from build123d import *

# Parameters (mm, degrees)
CROQUIS1_R              = 1.75
SALIENTE_EXTRUIR1_DEPTH = 2
CROQUIS2_R              = 1.75
SALIENTE_EXTRUIR2_DEPTH = 64
CORTAR_EXTRUIR1_DEPTH   = 62
REDONDEO1_R             = 2
CORTAR_EXTRUIR2_REACH   = 56
CROQUIS5_W              = 10.1
CROQUIS5_H              = 56.5


with BuildPart() as part:
    # Croquis1 → Saliente-Extruir1 (new body)
    with BuildSketch(Plane(origin=(0, 89.4998128, 0), x_dir=(1, 0, 0), z_dir=(0, 1, 0))):
        with BuildLine():
            Line((-45.118250968, 6.084971867), (-5.118250968, 6.084971867))
            ThreePointArc((-5.118250968, 6.084971867), (-0.1685035, 8.135224399), (1.881749032, 13.084971867))
            Line((1.881749032, 13.084971867), (1.881749032, 43.084971867))
            ThreePointArc((1.881749032, 43.084971867), (-0.1685035, 48.034719335), (-5.118250968, 50.084971867))
            Line((-5.118250968, 50.084971867), (-45.118250968, 50.084971867))
            ThreePointArc((-45.118250968, 50.084971867), (-50.067998436, 48.034719335), (-52.118250968, 43.084971867))
            Line((-52.118250968, 43.084971867), (-52.118250968, 13.084971867))
            ThreePointArc((-52.118250968, 13.084971867), (-50.067998436, 8.135224399), (-45.118250968, 6.084971867))
        make_face()
        with Locations((-48.118250968, 28.084971867)):
            Circle(CROQUIS1_R, mode=Mode.SUBTRACT)
        with Locations((-5.118250968, 43.084971867)):
            Circle(CROQUIS1_R, mode=Mode.SUBTRACT)
        with Locations((-5.118250968, 13.084971867)):
            Circle(CROQUIS1_R, mode=Mode.SUBTRACT)
        with BuildLine():
            Line((-45.118250968, 8.084971867), (-13.603532342, 8.084971867))
            ThreePointArc((-13.603532342, 8.084971867), (-11.97053918, 8.930271329), (-11.717914259, 10.751638534))
            ThreePointArc((-11.717914259, 10.751638534), (-11.945259003, 14.631568546), (-10.067998436, 18.034719335))
            Line((-10.067998436, 18.034719335), (-10.067998436, 38.135224399))
            ThreePointArc((-10.067998436, 38.135224399), (-11.945259003, 41.538375188), (-11.717914259, 45.4183052))
            ThreePointArc((-11.717914259, 45.4183052), (-11.97053918, 47.239672405), (-13.603532342, 48.084971867))
            Line((-13.603532342, 48.084971867), (-45.118250968, 48.084971867))
            ThreePointArc((-45.118250968, 48.084971867), (-48.653784874, 46.620505773), (-50.118250968, 43.084971867))
            Line((-50.118250968, 43.084971867), (-50.118250968, 37.084971867))
            ThreePointArc((-50.118250968, 37.084971867), (-49.53246453, 35.670758305), (-48.118250968, 35.084971867))
            ThreePointArc((-48.118250968, 35.084971867), (-41.118250968, 28.084971867), (-48.118250968, 21.084971867))
            ThreePointArc((-48.118250968, 21.084971867), (-49.53246453, 20.499185429), (-50.118250968, 19.084971867))
            Line((-50.118250968, 19.084971867), (-50.118250968, 13.084971867))
            ThreePointArc((-50.118250968, 13.084971867), (-48.653784874, 9.549437961), (-45.118250968, 8.084971867))
        make_face(mode=Mode.SUBTRACT)
    extrude(amount=SALIENTE_EXTRUIR1_DEPTH)

    # Croquis2 → Saliente-Extruir2 (add)
    with BuildSketch(Plane(origin=(0, 91.4998128, 0), x_dir=(1, 0, 0), z_dir=(0, 1, 0))):
        with BuildLine():
            Line((-45.118250968, 6.084971867), (-5.118250968, 6.084971867))
            ThreePointArc((-5.118250968, 6.084971867), (-0.1685035, 8.135224399), (1.881749032, 13.084971867))
            Line((1.881749032, 13.084971867), (1.881749032, 43.084971867))
            ThreePointArc((1.881749032, 43.084971867), (-0.1685035, 48.034719335), (-5.118250968, 50.084971867))
            Line((-5.118250968, 50.084971867), (-45.118250968, 50.084971867))
            ThreePointArc((-45.118250968, 50.084971867), (-50.067998436, 48.034719335), (-52.118250968, 43.084971867))
            Line((-52.118250968, 43.084971867), (-52.118250968, 13.084971867))
            ThreePointArc((-52.118250968, 13.084971867), (-50.067998436, 8.135224399), (-45.118250968, 6.084971867))
        make_face()
        with Locations((-48.118250968, 28.084971867)):
            Circle(CROQUIS2_R, mode=Mode.SUBTRACT)
        with Locations((-5.118250968, 43.084971867)):
            Circle(CROQUIS2_R, mode=Mode.SUBTRACT)
        with Locations((-5.118250968, 13.084971867)):
            Circle(CROQUIS2_R, mode=Mode.SUBTRACT)
        with BuildLine():
            Line((-10.067998436, 18.034719335), (-10.067998436, 38.135224399))
            ThreePointArc((-10.067998436, 38.135224399), (-11.945259003, 41.538375188), (-11.717914259, 45.4183052))
            ThreePointArc((-11.717914259, 45.4183052), (-11.97053918, 47.239672405), (-13.603532342, 48.084971867))
            Line((-13.603532342, 48.084971867), (-45.118250968, 48.084971867))
            ThreePointArc((-45.118250968, 48.084971867), (-48.653784874, 46.620505773), (-50.118250968, 43.084971867))
            Line((-50.118250968, 43.084971867), (-50.118250968, 37.084971867))
            ThreePointArc((-50.118250968, 37.084971867), (-49.53246453, 35.670758305), (-48.118250968, 35.084971867))
            ThreePointArc((-48.118250968, 35.084971867), (-41.118250968, 28.084971867), (-48.118250968, 21.084971867))
            ThreePointArc((-48.118250968, 21.084971867), (-49.53246453, 20.499185429), (-50.118250968, 19.084971867))
            Line((-50.118250968, 19.084971867), (-50.118250968, 13.084971867))
            ThreePointArc((-50.118250968, 13.084971867), (-48.653784874, 9.549437961), (-45.118250968, 8.084971867))
            Line((-45.118250968, 8.084971867), (-13.603532342, 8.084971867))
            ThreePointArc((-13.603532342, 8.084971867), (-11.97053918, 8.930271329), (-11.717914259, 10.751638534))
            ThreePointArc((-11.717914259, 10.751638534), (-11.945259003, 14.631568546), (-10.067998436, 18.034719335))
        make_face(mode=Mode.SUBTRACT)
    extrude(amount=SALIENTE_EXTRUIR2_DEPTH)

    # Croquis3 → Cortar-Extruir1 (cut)
    with BuildSketch(Plane(origin=(0, 155.4998128, 0), x_dir=(1, 0, 0), z_dir=(0, 1, 0))):
        with BuildLine():
            Line((-5.118250968, 38.084971867), (1.881749032, 38.084971867))
            Line((1.881749032, 38.084971867), (1.881749032, 43.084971867))
            ThreePointArc((1.881749032, 43.084971867), (-0.1685035, 48.034719335), (-5.118250968, 50.084971867))
            Line((-5.118250968, 50.084971867), (-13.603532342, 50.084971867))
            ThreePointArc((-13.603532342, 50.084971867), (-10.337546018, 48.394372944), (-9.832296176, 44.751638534))
            ThreePointArc((-9.832296176, 44.751638534), (-9.994685279, 41.980259953), (-8.653784874, 39.549437961))
            ThreePointArc((-8.653784874, 39.549437961), (-7.03166813, 38.465574204), (-5.118250968, 38.084971867))
        make_face()
        with BuildLine():
            Line((-5.118250968, 18.084971867), (1.881749032, 18.084971867))
            Line((1.881749032, 18.084971867), (1.881749032, 13.084971867))
            ThreePointArc((1.881749032, 13.084971867), (-0.1685035, 8.135224399), (-5.118250968, 6.084971867))
            Line((-5.118250968, 6.084971867), (-13.603532342, 6.084971867))
            ThreePointArc((-13.603532342, 6.084971867), (-10.337546018, 7.77557079), (-9.832296176, 11.4183052))
            ThreePointArc((-9.832296176, 11.4183052), (-9.994685279, 14.18968378), (-8.653784874, 16.620505773))
            ThreePointArc((-8.653784874, 16.620505773), (-7.03166813, 17.704369529), (-5.118250968, 18.084971867))
        make_face()
        with BuildLine():
            Line((-48.118250968, 23.084971867), (-52.118250968, 23.084971867))
            Line((-52.118250968, 23.084971867), (-52.118250968, 33.084971867))
            Line((-52.118250968, 33.084971867), (-48.118250968, 33.084971867))
            ThreePointArc((-48.118250968, 33.084971867), (-43.118250968, 28.084971867), (-48.118250968, 23.084971867))
        make_face()
    extrude(amount=-CORTAR_EXTRUIR1_DEPTH, mode=Mode.SUBTRACT)

    # Redondeo1
    redondeo1_edges = [part.edges().sort_by_distance(p)[0] for p in [
        (1.881749032, 124.4998128, -18.084971867),
        (1.881749032, 124.4998128, -38.084971867),
        (-52.118250968, 124.4998128, -23.084971867),
        (-52.118250968, 124.4998128, -33.084971867),
    ]]
    fillet(redondeo1_edges, radius=REDONDEO1_R)

    # Croquis5 → Cortar-Extruir2 (cut, up to next)
    with BuildSketch(Plane(origin=(1.881749032, 0, 0), x_dir=(0, 0, -1), z_dir=(1, 0, 0)), mode=Mode.PRIVATE) as cortar_extruir2_sk1:
        with Locations((28.084971867, 120.2498128)):
            Rectangle(CROQUIS5_W, CROQUIS5_H)
    cortar_extruir2_tool1 = extrude(cortar_extruir2_sk1.sketch, amount=-CORTAR_EXTRUIR2_REACH, mode=Mode.PRIVATE) & part.part
    add(cortar_extruir2_tool1.solids().sort_by_distance((1.881749, 120.249813, -28.084972))[0], mode=Mode.SUBTRACT)


solid = part.part
The listing builds one solid part. Answer for the finished solid, in the listing's coordinates (mm). A direction names the side the tool comes from. Coordinates: 2 decimals unless noted, no trailing zeros. Order: outer loops, then holes, each group sorted by start corner. A loop starts at its lowest first (then second) coordinate and runs counter-clockwise, first axis right, second up.
Q1. For a pull along X with two mould halves and no side action, classify faces 5 (the face through (-50.118, 122, -40)), 6 (the face through (1.882, 122, -22)), 7 (the face through (-50, 122, -48.1)), 8 (the face through (-49.55, 122.04, -35.69)) as pulls with the +X half, pulls with the -X half, needs draft (parallel to the pull), parting line crosses it, or undercut.
Q2. A cutting plane is placed at A-A, the plane x = -15. Write down the section's boundary in (y, z), and give its area (3 significant figures).
Q3. Consider line 1 (Z direction, x = -41, y = 95); line 2 (Z direction, x = -4, y = 135); line 3 (Z direction, x = -45, y = 126). Determine where each line is inside the solid, lowest interval first.
Q4. Which of the six approach directions +Z, -Z, +X, -X, +Y, -Y give full straight-line access (tool end or side, diameter ignored) to faces 1 (the face through (-10.37, 124.93, -7.73)), 2 (the face through (-29, 122, -48.085)), 3 (the face through (-3, 125, -38.085)), 4 (the face through (1.311, 124.066, -18.686))?
Q5. Given P1, Ø5.5, axis at x = -3, y = 112.5, coming from the +Z side; P2, Ø1, axis at y = 118.5, z = -25.5, coming from the +X side; P3, Ø3, axis at y = 146, z = -45.5, coming from the +X side, each flat-ended and moving along its own axis, determine where each tip first touches the part or whether it passes through.
Q6. A cutting plane is placed at B-B, the plane z = -25. Write down the section's boundary in (x, y), and give its area (3 significant figures).
Answers follow:
1. face 5: undercut
1. face 6: pulls with the +X half
1. face 7: pulls with the -X half
1. face 8: undercut
2. outline: (89.5, -50.08) - (155.5, -50.08) - (155.5, -48.08) - (89.5, -48.08) - close; (89.5, -8.08) - (155.5, -8.08) - (155.5, -6.08) - (89.5, -6.08) - close
2. area: 264 mm2
3. line 1: z = -50.08 to -48.08, -8.08 to -6.08
3. line 2: z = -38.08 to -33.13, -23.03 to -18.08
3. line 3: z = -50.08 to -48.08, -34.35 to -31.99, -24.18 to -21.82, -8.08 to -6.08
4. face 1: +X, +Y
4. face 2: +Y, -Y
4. face 3: -Z, +X, +Y
4. face 4: +Z, +X, +Y
5. P1: stops at z = -18.04
5. P2: stops at x = -41.44
5. P3: stops at x = -9.6
6. outline: (-52.12, 89.5) - (-41.83, 89.5) - (-41.83, 155.5) - (-44.18, 155.5) - (-44.18, 93.5) - (-52.12, 93.5) - close; (-10.07, 89.5) - (1.88, 89.5) - (1.88, 92) - (-10.07, 92) - close; (-10.07, 148.5) - (1.88, 148.5) - (1.88, 155.5) - (-10.07, 155.5) - close
6. area: 300 mm2
